Design review of the part built by this model. Coordinates are the model's own, in mm. A direction names the side the tool comes from. Coordinates: 2 decimals unless noted, no trailing zeros. Loops run counter-clockwise (first coordinate to the right, second up) from the corner with the lowest first, then second, coordinate; pieces in that order, holes last. Notation, with made-up numbers: M -26,29 L 0,29 A15 ccw 0,33 Z; hole C -20.75,-7.75 d3. An arc over 180 degrees is marked long. One line per item, written item: value.
```python
from build123d import *

# Parameters (mm, degrees)
SKETCH1_W                                = 20.746
SKETCH1_H                                = 24
BOSS_EXTRUDE1_DEPTH                      = 5.7
SKETCH9_W                                = 9.246
SKETCH9_H                                = 24
CUT_EXTRUDE3_DEPTH                       = 17.854943755
F_9_64_0_14063_DIAMETER_HOLE1_AT_2_COUNT = 2
F_9_64_0_14063_DIAMETER_HOLE1_AT_2_PITCH = 17
SKETCH8_R                                = 1.3
CUT_EXTRUDE2_DEPTH                       = 5.75
SKETCH10_W                               = 40.08
SKETCH10_H                               = 47.7
BOSS_EXTRUDE2_DEPTH                      = 2
SKETCH11_R                               = 2.515
BOSS_EXTRUDE3_DEPTH                      = 2
SKETCH12_R                               = 1
CUT_EXTRUDE4_DEPTH                       = 41.757486785
FILLET2_R                                = 2.5
CUT_EXTRUDE5_DEPTH                       = 40.994658756
FILLET3_R                                = 2.5
CUT_EXTRUDE6_DEPTH                       = 5.7


with BuildPart() as part:
    # Sketch1 → Boss-Extrude1 (new body)
    with BuildSketch(Plane(origin=(0, 0, 0), x_dir=(1, 0, 0), z_dir=(0, 1, 0))):
        Rectangle(SKETCH1_W, SKETCH1_H)
    extrude(amount=BOSS_EXTRUDE1_DEPTH)

    # Sketch9 → Cut-Extrude3 (cut, through all)
    with BuildSketch(Plane.XZ):
        Rectangle(SKETCH9_W, SKETCH9_H)
    extrude(amount=-CUT_EXTRUDE3_DEPTH, mode=Mode.SUBTRACT)


with BuildPart() as cut_extrude3_piece_1:
    # of the separate pieces the step leaves, piece 1, a body of its own (cut_extrude3_pieces)
    add(part.part.solids().sort_by_distance((-10.373, 0, -12))[0])

    # Sketch8 → Cut-Extrude2 (cut)
    with BuildSketch(Plane.ZY.offset(10.373)):
        with Locations((8, 2.9)):
            Circle(SKETCH8_R)
        with Locations((-9, 2.9)):
            Circle(SKETCH8_R)
    extrude(amount=-CUT_EXTRUDE2_DEPTH, mode=Mode.SUBTRACT)



with BuildPart() as cut_extrude3_piece_2:
    # of the separate pieces the step leaves, piece 2, a body of its own (cut_extrude3_pieces)
    add(part.part.solids().sort_by_distance((4.623, 0, -12))[0])

    # Sketch7 → 9/64 (0.14063) Diameter Hole1 (revolve, cut)
    with BuildSketch(Plane(origin=(10.373, 2.9, -9), x_dir=(0, 0, -1), z_dir=(0, 1, 0))):
        Polygon((0, 0), (0, 6.823137666), (1.786001, 5.75), (1.786001, 0), align=None)
    f_9_64_0_14063_diameter_hole1 = revolve(axis=Axis((16.723, 2.9, -9), (-1, 0, 0)), mode=Mode.SUBTRACT)

    # 9/64 (0.14063) Diameter Hole1 at 2: 9/64 (0.14063) Diameter Hole1 ×2
    with Locations(*[(0, 0, i * F_9_64_0_14063_DIAMETER_HOLE1_AT_2_PITCH) for i in range(1, F_9_64_0_14063_DIAMETER_HOLE1_AT_2_COUNT)]):
        add(f_9_64_0_14063_diameter_hole1, mode=Mode.SUBTRACT)


with BuildPart() as cut_extrude3_piece_1_1:
    add(cut_extrude3_piece_1.part)

    add(cut_extrude3_piece_2.part)  # Boss-Extrude2 merges Cut-Extrude3 piece 2
    # Sketch10 → Boss-Extrude2 (add)
    with BuildSketch(Plane.XZ):
        with Locations((-2.987, -8.35)):
            Rectangle(SKETCH10_W, SKETCH10_H)
    extrude(amount=BOSS_EXTRUDE2_DEPTH)

    # Sketch11 → Boss-Extrude3 (add)
    with BuildSketch(Plane.XZ.offset(2)):
        with Locations(Location((14.453, 12.9, 0), (0, 0, 90))):
            Circle(SKETCH11_R)
        with Locations(Location((-20.475, 12.985, 0), (0, 0, 90))):
            Circle(SKETCH11_R)
        with Locations(Location((14.45, -29.6362, 0), (0, 0, 90))):
            Circle(SKETCH11_R)
        with Locations(Location((-20.475, -29.6362, 0), (0, 0, 90))):
            Circle(SKETCH11_R)
    extrude(amount=BOSS_EXTRUDE3_DEPTH)

    # Sketch12 → Cut-Extrude4 (cut, through all)
    with BuildSketch(Plane.XZ.offset(4)):
        with Locations(Location((14.453, 12.9, 0), (0, 0, 270))):
            Circle(SKETCH12_R)
        with Locations(Location((-20.475, 12.985, 0), (0, 0, 270))):
            Circle(SKETCH12_R)
        with Locations(Location((-20.475, -29.6362, 0), (0, 0, 270))):
            Circle(SKETCH12_R)
        with Locations(Location((14.45, -29.6362, 0), (0, 0, 270))):
            Circle(SKETCH12_R)
    extrude(amount=-CUT_EXTRUDE4_DEPTH, mode=Mode.SUBTRACT)

    # Fillet2
    fillet2_edges = [cut_extrude3_piece_1_1.edges().sort_by_distance(p)[0] for p in [
        (17.053, -1, -32.2),
        (17.053, -1, 15.5),
        (-23.027, -1, 15.5),
        (-23.027, -1, -32.2),
    ]]
    fillet(fillet2_edges, radius=FILLET2_R)

    # Sketch14 → Cut-Extrude5 (cut, through all)
    with BuildSketch(Plane(origin=(0, 0, 0), x_dir=(1, 0, 0), z_dir=(0, 1, 0))):
        Polygon((10.553, 32.2), (10.553, 12), (-1.447, 12), (-8.799198732, 32.2), align=None)
    extrude(amount=-CUT_EXTRUDE5_DEPTH, mode=Mode.SUBTRACT)

    # Fillet3
    fillet3_edges = [cut_extrude3_piece_1_1.edges().sort_by_distance(p)[0] for p in [
        (10.553, -1, -12),
        (-1.447, -1, -12),
        (10.553, -1, -32.2),
        (-8.799198732, -1, -32.2),
    ]]
    fillet(fillet3_edges, radius=FILLET3_R)

    # Sketch15 → Cut-Extrude6 (cut)
    with BuildSketch(Plane(origin=(0, 5.7, 0), x_dir=(1, 0, 0), z_dir=(0, 1, 0))):
        with BuildLine():
            Line((8.053, 12), (10.373, 12))
            Line((10.373, 12), (10.373, 13.568549518))
            ThreePointArc((10.373, 13.568549518), (9.453245299, 12.428934308), (8.053, 12))
        make_face()
    extrude(amount=-CUT_EXTRUDE6_DEPTH, mode=Mode.SUBTRACT)


solid = cut_extrude3_piece_1_1.part
```
(1) We need section A-A on y = 2.9. State the section outline as (x, z) points, then the cut area to 3 significant figures.
Reply:
outline: M -10.37,-12 L -4.62,-12 L -4.62,-10.3 L -10.37,-10.3 Z; M -10.37,-7.7 L -4.62,-7.7 L -4.62,6.7 L -10.37,6.7 Z; M -10.37,9.3 L -4.62,9.3 L -4.62,12 L -10.37,12 Z; M 4.62,-12 L 10.37,-12 L 10.37,-10.79 L 4.62,-10.79 Z; M 4.62,-7.21 L 10.37,-7.21 L 10.37,6.21 L 4.62,6.21 Z; M 4.62,9.79 L 10.37,9.79 L 10.37,12 L 4.62,12 Z
area: 205 mm2
(2) We need section D-D on y = -2.75. State the section outline as (x, z) points (3 decimals).
Reply:
outline: C -20.475,-29.636 d5.03; C -20.475,12.985 d5.03; C 14.45,-29.636 d5.03; C 14.453,12.9 d5.03; hole C -20.475,-29.636 d2; hole C -20.475,12.985 d2; hole C 14.45,-29.636 d2; hole C 14.453,12.9 d2
(3) Tool access review of faces 1 (the flat face through (-8, 3, 12)), 2 (the flat face through (-10.373, 3, 0)), 3 (the flat face through (7, 2, -12)), 4 (the flat face through (10.373, 3, 0)), 5 (the cylindrical face through (11.305, -1.014, -31.487)): name each direction out of +Z, -Z, +X, -X, +Y, -Y from which nothing blocks a thin tool from reaching the whole face with its end or side.
Reply:
face 1: +Z, +X, -X, +Y
face 2: +Z, -Z, -X, +Y
face 3: -Z, +Y
face 4: +Z, -Z, +X, +Y
face 5: -Z, +Y, -Y
(4) We need section C-C on x = 5.5. State the section outline as (y, z) points, then the cut area to 3 significant figures.
Reply:
outline: M -2,-12 L 5.7,-12 L 5.7,12 L 0,12 L 0,15.5 L -2,15.5 Z; hole C 2.9,-9 d3.57; hole C 2.9,8 d3.57
area: 172 mm2
(5) We need section B-B on z = -9. State the section outline as (x, y) points.
Reply:
outline: M -23.03,-2 L 17.05,-2 L 17.05,0 L 10.37,0 L 10.37,1.11 L 4.62,1.11 L 4.62,0 L -4.62,0 L -4.62,1.6 L -10.37,1.6 L -10.37,0 L -23.03,0 Z; M -10.37,4.2 L -4.62,4.2 L -4.62,5.7 L -10.37,5.7 Z; M 4.62,4.69 L 10.37,4.69 L 10.37,5.7 L 4.62,5.7 Z
(6) Insertion check: pin 1 (3 mm diameter, centred on y = 3, z = -12, fed in from +X); pin 2 (1 mm diameter, centred on x = -12, z = 3, fed in from -Y); pin 3 (3 mm diameter, centred on y = 2.9, z = -9, fed in from +X); pin 4 (2.5 mm diameter, centred on x = -20.48, z = -29.64, fed in from -Y). Each pin has a flat end and moves straight along its axis. Give the tip position at first contact, or say it passes through.
Reply:
pin 1: stops at x = 10.37
pin 2: stops at y = -2
pin 3: stops at x = -4.62
pin 4: stops at y = -4
(7) Mouldability with a two-part tool opening along Y and no side actions: class faces 6 (the flat face through (16, -4, -30)), 7 (the flat face through (-8, 5.7, 0)), 8 (the cylindrical face through (7.54, 1.13, 8.23)), 9 (the flat face through (-8, 3, -12)) as released by +Y, released by -Y, zero draft, split by the parting line, or undercut.
Reply:
face 6: released by -Y
face 7: released by +Y
face 8: undercut
face 9: zero draft
(8) To check wall thickness, follow line 1 along Z through (x, y) = (8.75, 2.9); line 2 along X through (y, z) = (1.5, 10.5); line 3 along Y through (x, z) = (-6.9, -9). State the ranges of each line that lie inside material, in increasing order. Write a range as [from, to].
Reply:
line 1: z = [-12, -10.79], [-7.21, 6.21], [9.79, 12]
line 2: x = [-10.37, -4.62], [4.62, 10.37]
line 3: y = [-2, 1.6], [4.2, 5.7]
